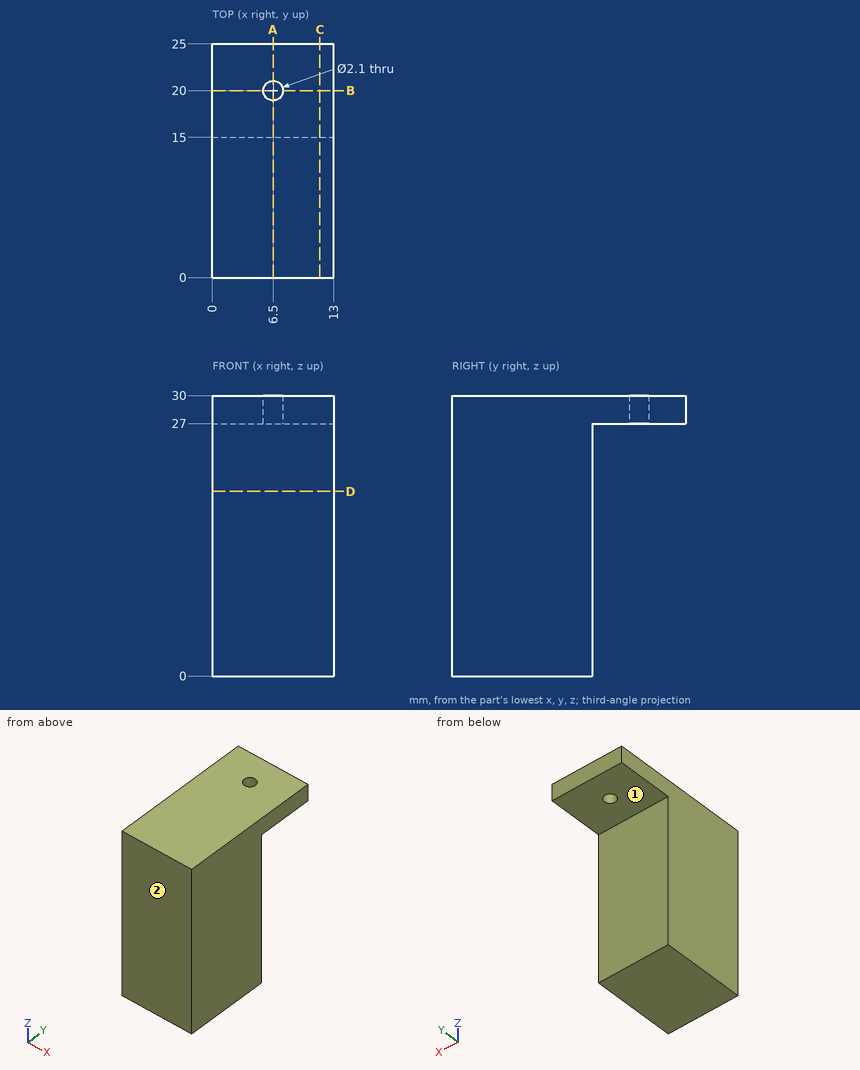
For this review, use the dimensioned drawing (mm, ordinates from the lowest corner) and the shaded views. A direction names the side the tool comes from. Round coordinates to 2 decimals unless told otherwise and drop trailing zeros. Write each loop counter-clockwise with the first axis right and the second up, starting at its lowest first coordinate (ties: lowest second). Pieces come first, ordered by that corner, then holes. Notation, with made-up numbers: (49.25, 88.25) - (94.25, 88.25) arc R23 cw to (94.25, 114.25) - close; hole circle Ø9 at (-32, 9). An arc over 180 degrees is marked (long way). Answer as CSV lines item,"result". Start each with the question number.
(1) We need section C-C on x = 11.5. State the section outline as (y, z) points.
(2) We need section D-D on z = 19.75. State the section outline as (x, y) points.
(3) For the marked faces 1 and 2, list the 3-axis set-ups (+Z, -Z, +X, -X, +Y, -Y) from which the entire face can be reached by the end or side of a thin tool; tool diameter is ignored.
(4) To check wall thickness, follow line 1 (Y direction, x = 6.5, z = 28.2); line 2 (Y direction, x = 6, z = 22); line 3 (Z direction, x = 1.5, y = 16). State the ranges of each line that lie inside material, in increasing order.
(5) We need section A-A on x = 6.5. State the section outline as (y, z) points.
(6) For pin 1 Ø1 at (x, z) = (4.5, 19) entering from +Y; pin 2 Ø5 at (x, y) = (8.5, 19.5) entering from -Z, all flat-tipped, find the tip position at first contact; note any pin that passes through.
(7) We need section B-B on y = 20. State the section outline as (x, z) points, plus the area to 3 significant figures.
Worked answers:
1,outline,"(0, 0) - (15, 0) - (15, 27) - (25, 27) - (25, 30) - (0, 30) - close"
2,outline,"(0, 0) - (13, 0) - (13, 15) - (0, 15) - close"
3,face 1,"-Z, +X, -X, +Y"
3,face 2,"+Z, -Z, +X, -X, -Y"
4,line 1,"0 to 18.95, 21.05 to 25"
4,line 2,"0 to 15"
4,line 3,"27 to 30"
5,outline,"(0, 0) - (15, 0) - (15, 27) - (18.95, 27) - (18.95, 30) - (0, 30) - close; (21.05, 27) - (25, 27) - (25, 30) - (21.05, 30) - close"
6,pin 1,"y = 15"
6,pin 2,"z = 27"
7,outline,"(0, 27) - (5.45, 27) - (5.45, 30) - (0, 30) - close; (7.55, 27) - (13, 27) - (13, 30) - (7.55, 30) - close"
7,area,"32.7 mm²"
